Part model, mm, in its own coordinate system. Face numbers are marked on the shaded views. Round coordinates to 2 decimals unless told otherwise and drop trailing zeros. Write each loop counter-clockwise with the first axis right and the second up, starting at its lowest first coordinate (ties: lowest second). Pieces come first, ordered by that corner, then holes. Notation, with made-up numbers: (-39.5, -38) -> (-7.5, -38) arc R10 ccw to (-7.5, -22) -> close; hole circle Ø8 at (84.5, 87.5). An arc over 180 degrees is marked (long way). Return JSON: item names as keys, results as strings. Group by question number.
(1) Drill centre lines: L1, parallel to X at y = 92, z = -6.35 (3 decimals); L2, parallel to Z at x = 6, y = 110.5; L3, parallel to X at y = 18.5, z = 31. Where is each one in solid material? Low to high. Write a range as from..to.
(2) Saw through at C-C (y = 36). List the corners of the cut face in (x, z) (3 decimals).
(3) Drop flat-ended pins along their axis: pin 1 Ø10 at (y, z) = (69.5, 29.5) entering from +X; pin 2 Ø6 at (x, y) = (-60, 87) entering from -Z; pin 3 Ø2 at (y, z) = (32, 46) entering from -X. Give the stop position or say it passes through.
(4) Mould opens along Z. For the marked faces 1, 2, 3 and 4 say: +Z half, -Z half, draft (parallel to the pull), parting line (faces both ways), or undercut.
(5) Saw through at B-B (x = 6.35). List the corners of the cut face in (y, z) (3 decimals).
(6) Saw through at A-A (z = -6.35). List the corners of the cut face in (x, y) (3 decimals).
from build123d import *

# Parameters (mm, degrees)
SKETCH1_W           = 12.7
SKETCH1_H           = 12.7
BOSS_EXTRUDE1_DEPTH = 12.7
SKETCH2_R           = 88.9
BOSS_EXTRUDE2_DEPTH = 101.6
SKETCH3_R           = 85.725
CUT_EXTRUDE1_DEPTH  = 96.52
SKETCH4_W           = 12.7
SKETCH4_H           = 12.7
CUT_EXTRUDE2_DEPTH  = 12.7
FILLET2_R           = 1.524


with BuildPart() as part:
    # Sketch1 → Boss-Extrude1 (new body)
    with BuildSketch(Plane(origin=(0, 0, 0), x_dir=(1, 0, 0), z_dir=(0, 1, 0))):
        with Locations((6.35, 6.35)):
            Rectangle(SKETCH1_W, SKETCH1_H)
    extrude(amount=BOSS_EXTRUDE1_DEPTH)

    # Sketch2 → Boss-Extrude2 (add)
    with BuildSketch(Plane(origin=(0, 12.7, 0), x_dir=(1, 0, 0), z_dir=(0, 1, 0))):
        with Locations(Location((6.35, 6.35, 0), (0, 0, 270))):
            Circle(SKETCH2_R)
    extrude(amount=BOSS_EXTRUDE2_DEPTH)

    # Sketch3 → Cut-Extrude1 (cut)
    with BuildSketch(Plane(origin=(0, 114.3, 0), x_dir=(1, 0, 0), z_dir=(0, 1, 0))):
        with Locations(Location((6.35, 6.35, 0), (0, 0, 270))):
            Circle(SKETCH3_R)
    extrude(amount=-CUT_EXTRUDE1_DEPTH, mode=Mode.SUBTRACT)

    # Sketch4 → Cut-Extrude2 (cut)
    with BuildSketch(Plane.XZ):
        with Locations((6.35, -6.35)):
            Rectangle(SKETCH4_W, SKETCH4_H)
    extrude(amount=-CUT_EXTRUDE2_DEPTH, mode=Mode.SUBTRACT)

    # Fillet2
    fillet2_edges = [part.edges().sort_by_distance(p)[0] for p in [
        (6.35, 114.3, -95.25),
        (6.35, 114.3, -92.075),
    ]]
    fillet(fillet2_edges, radius=FILLET2_R)


solid = part.part
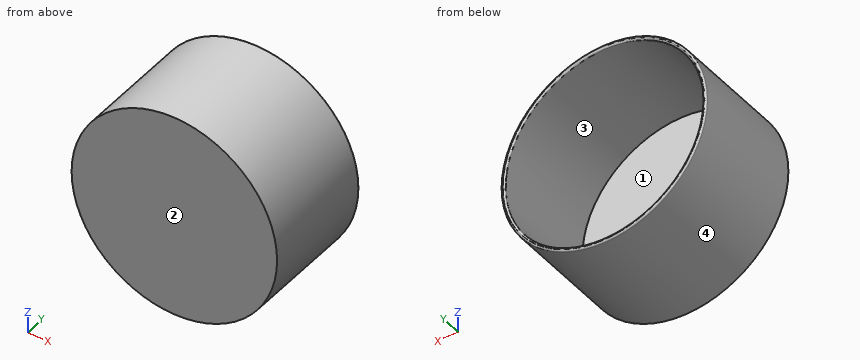
Computed values:
{
 "1": {"L1": "-82.55..-79.375, 92.075..95.25", "L2": "-95.25..-92.07, 79.37..82.55", "L3": "-74.32..-70.81, 83.51..87.02"},
 "2": {"outline": "circle Ø177.8 at (6.35, -6.35); hole circle Ø171.45 at (6.35, -6.35)"},
 "3": {"pin 1": "x = 89.73", "pin 2": "z = -68.72", "pin 3": "x = -66.22"},
 "4": {"face 1": "undercut", "face 2": "draft", "face 3": "undercut", "face 4": "parting line"},
 "5": {"outline": "(12.7, -95.25) -> (112.776, -95.25) arc R1.524 ccw to (114.3, -93.726) -> (114.3, -93.599) arc R1.524 ccw to (112.776, -92.075) -> (17.78, -92.075) -> (17.78, 79.375) -> (112.776, 79.375) arc R1.524 ccw to (114.3, 80.899) -> (114.3, 81.026) arc R1.524 ccw to (112.776, 82.55) -> (12.7, 82.55) -> close"},
 "6": {"outline": "(-82.55, 12.7) -> (95.25, 12.7) -> (95.25, 112.776) arc R1.524 ccw to (93.726, 114.3) -> (93.599, 114.3) arc R1.524 ccw to (92.075, 112.776) -> (92.075, 17.78) -> (-79.375, 17.78) -> (-79.375, 112.776) arc R1.524 ccw to (-80.899, 114.3) -> (-81.026, 114.3) arc R1.524 ccw to (-82.55, 112.776) -> close"}
}
